```python
from build123d import *

# Parameters (mm, degrees)
SKETCH_1_R      = 1.8
EXTRUDE_1_DEPTH = 7
SKETCH_2_R      = 1.8
EXTRUDE_2_DEPTH = 2
FILLET_1_R      = 0.4


with BuildPart() as part:
    # 草图1 → 凸台-拉伸1 (new body)
    with BuildSketch(Plane.XY):
        with BuildLine():
            Line((-0.405379361, 8.506127058), (-11.987060741, -4.413883456))
            ThreePointArc((-11.987060741, -4.413883456), (-12.07878067, -4.999252001), (-11.58168138, -5.321682108))
            Line((-11.58168138, -5.321682108), (-6.605215139, -5.321682108))
            Line((-6.605215139, -5.321682108), (-6.605215139, -8.142739227))
            ThreePointArc((-6.605215139, -8.142739227), (-6.445283211, -8.528172909), (-6.059454045, -8.687148374))
            Line((-6.059454045, -8.687148374), (0, -8.672119378))
            Line((0, -8.672119378), (6.059454045, -8.687148374))
            ThreePointArc((6.059454045, -8.687148374), (6.445283211, -8.528172909), (6.605215139, -8.142739227))
            Line((6.605215139, -8.142739227), (6.605215139, -5.321682108))
            Line((6.605215139, -5.321682108), (11.58168138, -5.321682108))
            ThreePointArc((11.58168138, -5.321682108), (12.07878067, -4.999252001), (11.987060741, -4.413883456))
            Line((11.987060741, -4.413883456), (0.405379361, 8.506127058))
            ThreePointArc((0.405379361, 8.506127058), (0, 8.687150048), (-0.405379361, 8.506127058))
        make_face()
        with Locations((0, -1.308282587)):
            Circle(SKETCH_1_R, mode=Mode.SUBTRACT)
    extrude(amount=EXTRUDE_1_DEPTH)

    # 草图2 → 凸台-拉伸2 (add)
    with BuildSketch(Plane(origin=(0, 0, 0), x_dir=(-1, 0, 0), z_dir=(0, 0, -1))):
        with Locations((0, -1.308282587)):
            Circle(SKETCH_2_R)
    extrude(amount=-EXTRUDE_2_DEPTH)

    # 圆角1
    fillet_1_edges = [part.edges().sort_by_distance(p)[0] for p in [
        (6.196220051, 2.046121801, 0),
        (12.07878067, -4.999252001, 0),
        (9.09344826, -5.321682108, 0),
        (6.605215139, -6.732210668, 0),
        (6.445283211, -8.528172909, 0),
        (3.029727022, -8.679633876, 0),
        (-3.029727022, -8.679633876, 0),
        (-6.445283211, -8.528172909, 0),
        (-6.605215139, -6.732210668, 0),
        (-9.09344826, -5.321682108, 0),
        (-12.07878067, -4.999252001, 0),
        (-6.196220051, 2.046121801, 0),
        (0, 8.687150048, 0),
    ]]
    fillet(fillet_1_edges, radius=FILLET_1_R)


solid = part.part
```
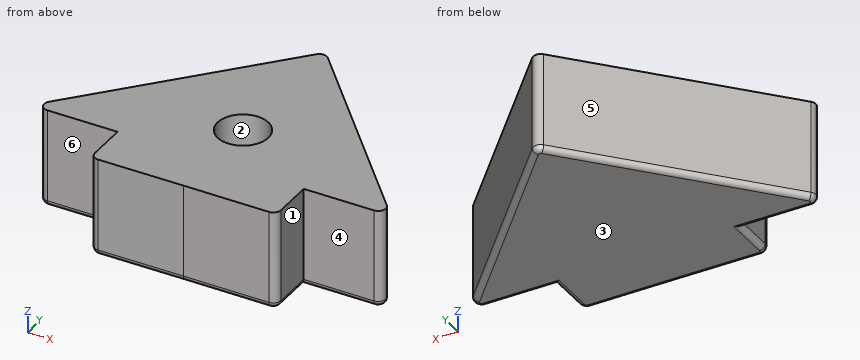
Here's how the part is built. I have some questions about the finished solid (model axes, mm). Face numbers are marked on the shaded views. A direction names the side the tool comes from. Round coordinates to 2 decimals unless told otherwise and drop trailing zeros. Loops run counter-clockwise (first coordinate to the right, second up) from the corner with the lowest first, then second, coordinate; pieces in that order, holes last. Notation, with made-up numbers: (-8, -28) -> (7, -28) arc R20 cw to (7, -2) -> close; hole circle Ø9 at (12, -13.75). An arc over 180 degrees is marked (long way). Answer as CSV lines item,"result". Start each with the question number.
1. For the marked faces 4, 5 and 6, which set-ups out of +Z, -Z, +X, -X, +Y, -Y let a thin tool reach every point of the face, with its end or its side?
2. I'm going to push flat-ended pins straight in: P1, Ø1.5, axis at x = 10.5, z = 3, coming from the -Y side; P2, Ø1.1, axis at x = 1, y = -1, coming from the +Z side; P3, Ø3, axis at x = 0, z = 2.5, coming from the -Y side. Where does each tip first touch, or does it pass through?
3. Imagine slicing it at A-A on y = -5.75. Write out the boundary of the cut face in (x, z), plus the area to 3 significant figures.
4. Imagine slicing it at C-C on z = 6. Write out the boundary of the cut face in (x, y), plus the area to 3 significant figures.
5. If we mould it in two halves opening along X, with no side actions, what happens to the marked faces 1, 2 and 3? For each: pulls with the +X half, pulls with the -X half, needs draft (parallel to the pull), parting line crosses it, or undercut.
6. Imagine slicing it at B-B on z = 1.75. Write out the boundary of the cut face in (x, y).
7. I need wall thicknesses on probe 1 along Y at (x, z) = (0, 3.45); probe 2 along X at (y, z) = (-6.5, 4.5); probe 3 along X at (y, z) = (0, 2.25). Which ranges of each line are inside material? Lowest first, please. Write a range as from..to.
Solution:
1,face 4,"+Z, -Z, +X, -Y"
1,face 5,"+Z, -Z, -X, +Y"
1,face 6,"+Z, -Z, -X, -Y"
2,P1,"y = -5.32"
2,P2,"z = 2"
2,P3,"y = -8.68"
3,outline,"(-6.61, 0.4) arc R0.4 ccw to (-6.21, 0) -> (6.21, 0) arc R0.4 ccw to (6.61, 0.4) -> (6.61, 7) -> (-6.61, 7) -> close"
3,area,"92.4 mm²"
4,outline,"(-11.99, -4.41) arc R0.54 ccw to (-11.58, -5.32) -> (-6.61, -5.32) -> (-6.61, -8.14) arc R0.54 ccw to (-6.06, -8.69) -> (0, -8.67) -> (6.06, -8.69) arc R0.54 ccw to (6.61, -8.14) -> (6.61, -5.32) -> (11.58, -5.32) arc R0.54 ccw to (11.99, -4.41) -> (0.41, 8.51) arc R0.54 ccw to (-0.41, 8.51) -> close; hole circle Ø3.6 at (0, -1.31)"
4,area,"216 mm²"
5,face 1,"pulls with the +X half"
5,face 2,"undercut"
5,face 3,"needs draft"
6,outline,"(-11.99, -4.41) arc R0.54 ccw to (-11.58, -5.32) -> (-6.61, -5.32) -> (-6.61, -8.14) arc R0.54 ccw to (-6.06, -8.69) -> (0, -8.67) -> (6.06, -8.69) arc R0.54 ccw to (6.61, -8.14) -> (6.61, -5.32) -> (11.58, -5.32) arc R0.54 ccw to (11.99, -4.41) -> (0.41, 8.51) arc R0.54 ccw to (-0.41, 8.51) -> close"
7,probe 1,"-8.67..-3.11, 0.49..8.69"
7,probe 2,"-6.61..6.61"
7,probe 3,"-8.03..-1.24, 1.24..8.03"
